Design review of the part built by this model. Coordinates are the model's own, in mm. Give positions to 0.01 mm unless a question says otherwise; leave off trailing zeros. Loops run counter-clockwise (first coordinate to the right, second up) from the corner with the lowest first, then second, coordinate; pieces in that order, holes last.
from build123d import *

# Parameters (mm, degrees)
SKETCH1_W           = 86
SKETCH1_H           = 60
BOSS_EXTRUDE1_DEPTH = 3
SKETCH4_W           = 45
SKETCH4_H           = 3
BOSS_EXTRUDE2_DEPTH = 35
SKETCH2_W           = 3
SKETCH2_H           = 5
CUT_EXTRUDE1_DEPTH  = 3
SKETCH8_W           = 3
SKETCH8_H           = 5
CUT_EXTRUDE10_DEPTH = 4
LPATTERN3_COUNT     = 2
LPATTERN3_PITCH     = 35
FILLET1_R           = 5
LPATTERN1_COUNT     = 3
LPATTERN1_PITCH     = 35
SKETCH5_R           = 1.5
CUT_EXTRUDE2_DEPTH  = 4
SKETCH6_R           = 3
CUT_EXTRUDE3_DEPTH  = 4


with BuildPart() as part:
    # Sketch1 → Boss-Extrude1 (new body)
    with BuildSketch(Plane(origin=(0, 0, 0), x_dir=(1, 0, 0), z_dir=(0, 1, 0))):
        with Locations((43, 30)):
            Rectangle(SKETCH1_W, SKETCH1_H)
    extrude(amount=BOSS_EXTRUDE1_DEPTH)

    # Sketch4 → Boss-Extrude2 (add)
    with BuildSketch(Plane(origin=(0, 0, -60), x_dir=(-1, 0, 0), z_dir=(0, 0, -1))):
        with Locations((-63.5, 1.5)):
            Rectangle(SKETCH4_W, SKETCH4_H)
    extrude(amount=BOSS_EXTRUDE2_DEPTH)

    # Sketch2 → Cut-Extrude1 (cut)
    with BuildSketch(Plane(origin=(0, 3, 0), x_dir=(1, 0, 0), z_dir=(0, 1, 0))):
        with Locations((63.5, 12.5)):
            Rectangle(SKETCH2_W, SKETCH2_H)
        with Locations((47.5, 12.5)):
            Rectangle(SKETCH2_W, SKETCH2_H)
        with Locations((81.3, 12.5)):
            Rectangle(SKETCH2_W, SKETCH2_H)
    cut_extrude1 = extrude(amount=-CUT_EXTRUDE1_DEPTH, mode=Mode.SUBTRACT)

    # Sketch8 → Cut-Extrude10 (cut, through all)
    with BuildSketch(Plane(origin=(0, 3, 0), x_dir=(1, 0, 0), z_dir=(0, 1, 0))):
        with Locations((6.5, 12.5)):
            Rectangle(SKETCH8_W, SKETCH8_H)
        with Locations((27.5, 12.5)):
            Rectangle(SKETCH8_W, SKETCH8_H)
    cut_extrude10 = extrude(amount=-CUT_EXTRUDE10_DEPTH, mode=Mode.SUBTRACT)

    # LPattern3: Cut-Extrude10 ×2
    with Locations(*[(0, 0, -i * LPATTERN3_PITCH) for i in range(1, LPATTERN3_COUNT)]):
        add(cut_extrude10, mode=Mode.SUBTRACT)

    # Fillet1
    fillet1_edges = [part.edges().sort_by_distance(p)[0] for p in [
        (41, 1.5, -60),
        (86, 1.5, -95),
        (41, 1.5, -95),
        (0, 1.5, -60),
        (86, 1.5, 0),
        (0, 1.5, 0),
    ]]
    fillet(fillet1_edges, radius=FILLET1_R)

    # LPattern1: Cut-Extrude1 ×3
    with Locations(*[(0, 0, -i * LPATTERN1_PITCH) for i in range(1, LPATTERN1_COUNT)]):
        add(cut_extrude1, mode=Mode.SUBTRACT)

    # Sketch5 → Cut-Extrude2 (cut, through all)
    with BuildSketch(Plane(origin=(0, 3, 0), x_dir=(1, 0, 0), z_dir=(0, 1, 0))):
        with Locations((17, 12.5)):
            Circle(SKETCH5_R)
        with Locations((17, 47.5)):
            Circle(SKETCH5_R)
        with Locations((72.5, 12.5)):
            Circle(SKETCH5_R)
        with Locations((55.5, 82.5)):
            Circle(SKETCH5_R)
    extrude(amount=-CUT_EXTRUDE2_DEPTH, mode=Mode.SUBTRACT)

    # Sketch6 → Cut-Extrude3 (cut, through all)
    with BuildSketch(Plane(origin=(0, 3, 0), x_dir=(1, 0, 0), z_dir=(0, 1, 0))):
        with Locations((34, 12.5)):
            Circle(SKETCH6_R)
        with Locations((34, 47.5)):
            Circle(SKETCH6_R)
    extrude(amount=-CUT_EXTRUDE3_DEPTH, mode=Mode.SUBTRACT)


solid = part.part
Q1. Take a section at C-C (z = -47.5). Give the number of separate pieces and of enclosed holes in the cut face, plus the area to 3 significant figures.
Results:
separate pieces: 8
enclosed holes: 0
area: 186 mm2
Q2. Draft analysis for pull direction Z (two halves, no side actions). For faces 1 (the face through (81, 2, -10)), 2 (the face through (20, 1, -60)), 3 (the face through (41, 1, -77)), state which applies: pulls with the +Z half, pulls with the -Z half, needs draft (parallel to the pull), parting line crosses it, or undercut.
Results:
face 1: undercut
face 2: pulls with the -Z half
face 3: needs draft
Q3. Take a section at B-B (x = 17). Give the boundary of the cut face in (y, z).
Results:
outline: (0, -60) - (3, -60) - (3, -49) - (0, -49) - close; (0, -46) - (3, -46) - (3, -14) - (0, -14) - close; (0, -11) - (3, -11) - (3, 0) - (0, 0) - close
Q4. Insertion check: pin 1 (5 mm diameter, centred on x = 17, z = -12.5, fed in from +Y); pin 2 (0.9 mm diameter, centred on x = 27, y = 1.5, fed in from -Z). Each pin has a flat end and moves straight along its axis. Give the tip position at first contact, or say it passes through.
Results:
pin 1: stops at y = 3
pin 2: stops at z = -60
Q5. Take a section at A-A (z = -82.5). Give the boundary of the cut face in (x, y), plus the area to 3 significant figures.
Results:
outline: (41, 0) - (46, 0) - (46, 3) - (41, 3) - close; (49, 0) - (54, 0) - (54, 3) - (49, 3) - close; (57, 0) - (62, 0) - (62, 3) - (57, 3) - close; (65, 0) - (79.8, 0) - (79.8, 3) - (65, 3) - close; (82.8, 0) - (86, 0) - (86, 3) - (82.8, 3) - close
area: 99.0 mm2
Q6. Wall thickness on line 1 (Z direction, x = 27, y = 1); line 2 (Z direction, x = 48.5, y = 0.35); line 3 (X direction, y = 1.6, z = -82.5): over which ranges is each line inside the solid? List them lowest first.
Results:
line 1: z = -60 to -50, -45 to -15, -10 to 0
line 2: z = -95 to -85, -80 to -50, -45 to -15, -10 to 0
line 3: x = 41 to 46, 49 to 54, 57 to 62, 65 to 79.8, 82.8 to 86
